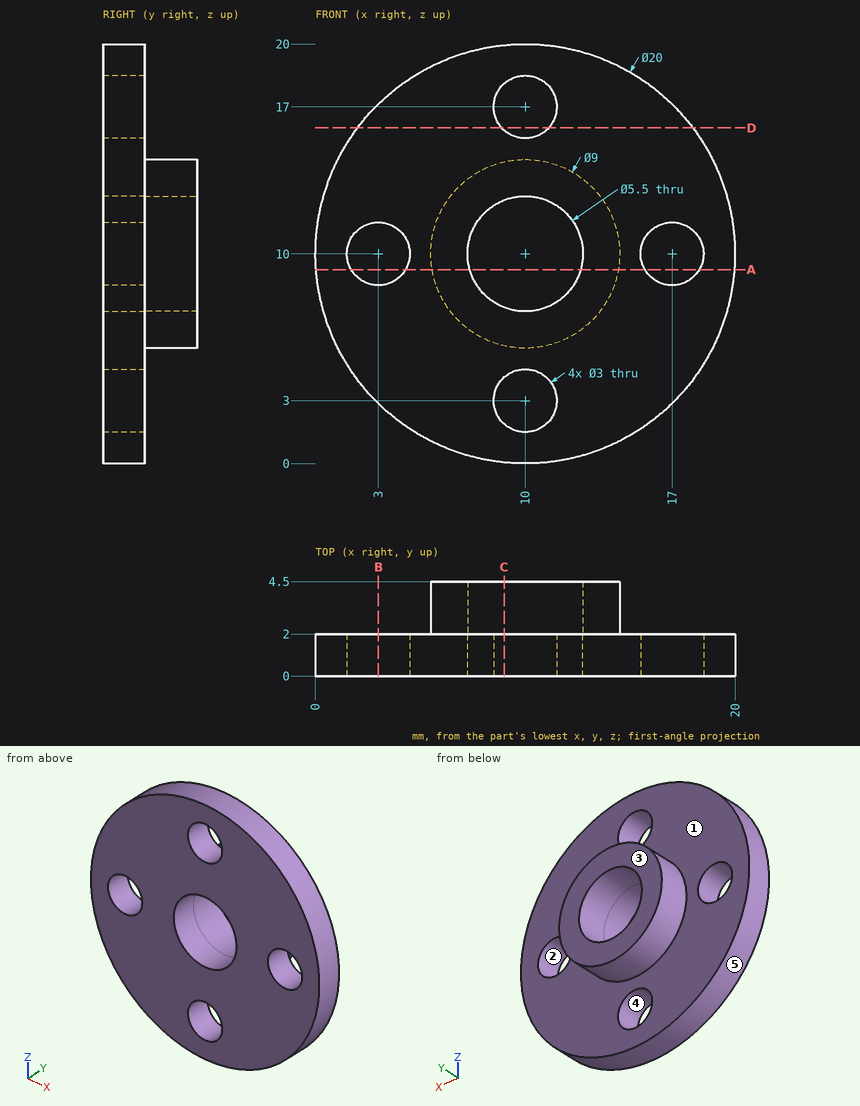
Input: dimensioned drawing with shaded views. Units: mm. Origin: part minimum x, y, z. A direction names the side the tool comes from. Give positions to 0.01 mm unless a question says otherwise; leave off trailing zeros. Order: outer loops, then holes, each group sorted by start corner. A loop starts at its lowest first (then second) coordinate and runs counter-clockwise, first axis right, second up. Notation, with made-up numbers: (72.5, 0.5) -> (93.5, 0.5) arc R10 ccw to (93.5, 8.5) -> close; hole circle Ø3 at (-2, 9.5). An arc over 180 degrees is marked (long way). Answer as a JSON object with one key per item and string values.
Q1. Access query for the marked faces 1 and 2. Directions: +Z, -Z, +X, -X, +Y, -Y. A direction counts if a zero-diameter tool reaches every point of the face in a straight line with its end or side. Return the directions, or none.
Entries:
{"face 1": "+Y", "face 2": "+Y, -Y"}
Q2. Section A-A (z = 9.25). Output: boundary loops of the cut face in (x, y).
Entries:
{"outline": "(0.03, 0) -> (1.7, 0) -> (1.7, 2) -> (0.03, 2) -> close; (4.3, 0) -> (7.35, 0) -> (7.35, 4.5) -> (5.56, 4.5) -> (5.56, 2) -> (4.3, 2) -> close; (12.65, 0) -> (15.7, 0) -> (15.7, 2) -> (14.44, 2) -> (14.44, 4.5) -> (12.65, 4.5) -> close; (18.3, 0) -> (19.97, 0) -> (19.97, 2) -> (18.3, 2) -> close"}
Q3. Draft query along Z for the marked faces 3, 4 and 5. Return one class per face: released by +Z, released by -Z, zero draft, split by the parting line, or undercut.
Entries:
{"face 3": "zero draft", "face 4": "undercut", "face 5": "split by the parting line"}
Q4. Section B-B (x = 3). Output: boundary loops of the cut face in (y, z).
Entries:
{"outline": "(0, 2.86) -> (2, 2.86) -> (2, 8.5) -> (0, 8.5) -> close; (0, 11.5) -> (2, 11.5) -> (2, 17.14) -> (0, 17.14) -> close"}
Q5. Section D-D (z = 16). Output: boundary loops of the cut face in (x, y), plus the area to 3 significant figures.
Entries:
{"outline": "(2, 0) -> (8.88, 0) -> (8.88, 2) -> (2, 2) -> close; (11.12, 0) -> (18, 0) -> (18, 2) -> (11.12, 2) -> close", "area": "27.5 mm^2"}
Q6. First-contact query: pin 1 (6 mm diameter, centred on x = 3.5, z = 5.5, fed in from -Y); pin 2 (3.5 mm diameter, centred on x = 10, z = 17, fed in from +Y). Flat tips, straight axial feed; report the tip coordinate or a pass-through.
Entries:
{"pin 1": "stops at y = 0", "pin 2": "stops at y = 2"}
Q7. Section C-C (x = 9). Output: boundary loops of the cut face in (y, z).
Entries:
{"outline": "(0, 0.05) -> (2, 0.05) -> (2, 1.88) -> (0, 1.88) -> close; (0, 4.12) -> (2, 4.12) -> (2, 5.61) -> (4.5, 5.61) -> (4.5, 7.44) -> (0, 7.44) -> close; (0, 12.56) -> (4.5, 12.56) -> (4.5, 14.39) -> (2, 14.39) -> (2, 15.88) -> (0, 15.88) -> close; (0, 18.12) -> (2, 18.12) -> (2, 19.95) -> (0, 19.95) -> close"}
Q8. Material intervals for probe 1 along Y at (x, z) = (13.5, 14); probe 2 along X at (y, z) = (1.1, 3); probe 3 along Z at (x, y) = (10.75, 2.3), sorted ascending.
Entries:
{"probe 1": "y = 0 to 2", "probe 2": "x = 2.86 to 8.5, 11.5 to 17.14", "probe 3": "z = 5.56 to 7.35, 12.65 to 14.44"}
